from build123d import *

# Parameters (mm, degrees)
F0_W      = 250
F0_H      = 200
F1_DEPTH  = 40
F3_DEPTH  = 18
F4_R      = 21
F5_DEPTH  = 10
F6_W      = 12
F6_H      = 73
F7_DEPTH  = 25
F8_W      = 155
F8_H      = 15
F9_DEPTH  = 25
F9_FACE_W = 155
F9_FACE_H = 25
F10_DEPTH = 47


with BuildPart() as f1:
    # F0 (on Top) → F1 (new body)
    with BuildSketch(Plane.XY):
        with Locations((-49.009792, 13.782904)):
            Rectangle(F0_W, F0_H)
    extrude(amount=F1_DEPTH)

    # F2 (on face) → F3 (cut)
    with BuildSketch(Plane.XY.offset(40)):
        with BuildLine():
            ThreePointArc((-151.139951, -29.209269), (-135.639951, -44.709269), (-120.139951, -29.209269))
            Line((-120.139951, -29.209269), (-120.139951, 62.790731))
            ThreePointArc((-120.139951, 62.790731), (-135.639951, 78.290731), (-151.139951, 62.790731))
            Line((-151.139951, 62.790731), (-151.139951, -29.209269))
        make_face()
    extrude(amount=-F3_DEPTH, mode=Mode.SUBTRACT)

    # F4 (on face) → F5 (cut)
    with BuildSketch(Plane.XY.offset(40)):
        with Locations((-88.571906, 0)):
            Circle(F4_R)
    extrude(amount=-F5_DEPTH, mode=Mode.SUBTRACT)

    # F6 (on face) → F7 (cut)
    with BuildSketch(Plane.XY.offset(40)):
        with Locations((-44.527275, 11.491382)):
            Rectangle(F6_W, F6_H)
    extrude(amount=-F7_DEPTH, mode=Mode.SUBTRACT)

    # F8 (on face) → F9 (join)
    with BuildSketch(Plane.XY.offset(40)):
        with Locations((-47.150943, 102.282946)):
            Rectangle(F8_W, F8_H)
    extrude(amount=F9_DEPTH)

    # F9_face (on face) → F10 (cut)
    with BuildSketch(Plane(origin=(-47.150943, 94.782946, 52.5), x_dir=(1, 0, 0), z_dir=(0, -1, 0))):
        Rectangle(F9_FACE_W, F9_FACE_H)
    extrude(amount=-F10_DEPTH, mode=Mode.SUBTRACT)


solid = f1.part
Model file for the job. Use its own axes, mm. A direction names the side the tool comes from. Round coordinates to 2 decimals unless told otherwise and drop trailing zeros. Order: outer loops, then holes, each group sorted by start corner. A loop starts at its lowest first (then second) coordinate and runs counter-clockwise, first axis right, second up. Notation, with made-up numbers: M 4.25,-36 L 46.25,-36 A32 cw 46.25,-1 Z; hole C 19,14.25 d3. An arc over 180 degrees is marked long. Write each question's results on one line, items separated by ' | '. Start each with the question number.
(1) Saw through at C-C, the plane y = 0. Give the cut face in (x, z).
(2) Two-plate mould, pull along X, no slides. Class faces 3 (the face through (-51, 15, 0)), 4 (the face through (-135.981, -44.706, 31.126)), 5 (the face through (-174.01, 12, 20)): pulls with the +X half, pulls with the -X half, needs draft (parallel to the pull), parting line crosses it, or undercut.
(3) Which spindle directions (+Z, -Z, +X, -X, +Y, -Y) get a long thin tool onto all of the face, cutting with end or side? Do faces 1 (the face through (-51, -86.217, 20)), 2 (the face through (-45, 12, 15)). Say none if no direction does.
(4) Saw through at D-D, the plane y = 52.5. Give the cut face in (x, z), then the cut area to 3 significant figures.
(5) Drop flat-ended pins along their axis: pin 1 (6 mm diameter, centred on x = -47, y = 7, fed in from +Z); pin 2 (1 mm diameter, centred on x = -88, y = 3.5, fed in from +Z); pin 3 (25 mm diameter, centred on x = -137.5, y = 4, fed in from +Z). Give the stop position or say it passes through.
(6) Probe probe 1 along X at (y, z) = (24, 29); probe 2 along X at (y, z) = (58, 38.5); probe 3 along Z at (x, y) = (-40.5, -24.5). List the from-to ranges inside material, lowest first. Write a range as from..to.
(7) Saw through at A-A, the plane z = 34.5. Give the cut face in (x, y).
(8) Saw through at B-B, the plane y = 24.5. Give the cut face in (x, z), then the cut area to 3 significant figures.
Established:
1) outline: M -174.01,0 L 75.99,0 L 75.99,40 L -38.53,40 L -38.53,15 L -50.53,15 L -50.53,40 L -67.57,40 L -67.57,30 L -109.57,30 L -109.57,40 L -120.14,40 L -120.14,22 L -151.14,22 L -151.14,40 L -174.01,40 Z
2) face 3: needs draft | face 4: undercut | face 5: pulls with the -X half
3) face 1: +Z, -Z, +X, -X, -Y | face 2: +Z
4) outline: M -174.01,0 L 75.99,0 L 75.99,40 L -120.14,40 L -120.14,22 L -151.14,22 L -151.14,40 L -174.01,40 Z | area: 9,440 mm^2
5) pin 1: stops at z = 15 | pin 2: stops at z = 30 | pin 3: stops at z = 22
6) probe 1: x = -174.01..-151.14, -120.14..-50.53, -38.53..75.99 | probe 2: x = -174.01..-151.14, -120.14..75.99 | probe 3: z = 0..15
7) outline: M -174.01,-86.22 L 75.99,-86.22 L 75.99,113.78 L -174.01,113.78 Z; hole M -151.14,-29.21 A15.5 ccw -120.14,-29.21 L -120.14,62.79 A15.5 ccw -151.14,62.79 Z; hole C -88.57,0 d42; hole M -50.53,-25.01 L -38.53,-25.01 L -38.53,47.99 L -50.53,47.99 Z
8) outline: M -174.01,0 L 75.99,0 L 75.99,40 L -38.53,40 L -38.53,15 L -50.53,15 L -50.53,40 L -120.14,40 L -120.14,22 L -151.14,22 L -151.14,40 L -174.01,40 Z | area: 9,140 mm^2
